Check sheet for the modelled part. Datum: model origin and axes. Units: mm. A direction names the side the tool comes from. Give positions to 0.01 mm unless a question says otherwise; leave off trailing zeros. Write each loop counter-clockwise with the first axis right and the second up, starting at its lowest first coordinate (ties: lowest second). Pieces come first, ordered by that corner, then holes. Notation, with made-up numbers: M 44.5,65 L 66.5,65 A22 ccw 66.5,101 Z; hole C 82.25,-35.5 d2. An arc over 180 degrees is marked long. Use CSV: the item, a comma, the result in double quotes. Start each with the question number.
1. Cross-section at C-C, the plane x = 3. Enter the section's corners in (y, z), and give its area (3 significant figures).
2. Depth check by flat-ended pin: P1, Ø3, axis at y = 15.5, z = 50.5, coming from the +X side (3 decimals); P2, Ø1, axis at x = 95.5, y = -12, coming from the +Z side; P3, Ø15, axis at y = -21, z = 38, coming from the -X side; P4, Ø5, axis at y = -3, z = 22.5, coming from the +X side. Enter the tip coordinate at first touch or a pass-through.
3. Scan lines: line 1 (Y direction, x = 46, z = 8); line 2 (Z direction, x = 12, y = -21); line 3 (X direction, y = -26, z = 47). Record each from-to range of solid material in increasing order.
4. Cross-section at A-A, the plane y = -21. Enter the section's corners in (x, z).
5. Mould release check, pull along Y, two halves, no side actions. Record for faces 1 (the face through (0, -21, 28)), 2 (the face through (36.5, -20.8, 9.6)), 3 (the face through (32, -42, 10)): +Y half, -Y half, draft (parallel to the pull), parting line (faces both ways), or undercut.
6. Cross-section at D-D, the plane z = 7. Enter the section's corners in (x, y), and give its area (3 significant figures).
7. Cross-section at B-B, the plane z = 39.5. Enter the section's corners in (x, y), and give its area (3 significant figures).
8. Access from +Z, -Z, +X, -X, +Y, -Y to the whole of each face (thin tool, end or side, straight path). Record for faces 4 (the face through (-6.8, 10.8, 32.1)), 5 (the face through (56.978, 10.846, 31.805)), 6 (the face through (65, -29, 19)).
from build123d import *

# Parameters (mm, degrees)
F0_W      = 42
F0_H      = 16
F1_DEPTH  = 112
F2_W      = 42
F2_H      = 22
F3_DEPTH  = 22
F4_R      = 9.5
F5_DEPTH  = 25
F6_W      = 42
F6_H      = 16
F7_DEPTH  = 21
F9_DEPTH  = 3
F11_DEPTH = 58
F13_DEPTH = 54
F15_DEPTH = 22


with BuildPart() as f1:
    # F0 (on Right) → F1 (new body)
    with BuildSketch(Plane.YZ):
        with Locations((-21, 8)):
            Rectangle(F0_W, F0_H)
    extrude(amount=F1_DEPTH)

    # F2 (on face) → F3 (join)
    with BuildSketch(Plane(origin=(0, 0, 0), x_dir=(0, -1, 0), z_dir=(-1, 0, 0))):
        with Locations((21, 27)):
            Rectangle(F2_W, F2_H)
        with BuildLine():
            ThreePointArc((42, 38), (21, 59), (0, 38))
            Line((0, 38), (42, 38))
        make_face()
    extrude(amount=-F3_DEPTH)

    # F4 (on face) → F5 (cut)
    with BuildSketch(Plane(origin=(0, 0, 0), x_dir=(0, -1, 0), z_dir=(-1, 0, 0))):
        with Locations((21, 38)):
            Circle(F4_R)
    extrude(amount=-F5_DEPTH, mode=Mode.SUBTRACT)

    # F6 (on face) → F7 (join)
    with BuildSketch(Plane(origin=(0, 0, 0), x_dir=(0, -1, 0), z_dir=(-1, 0, 0))):
        with Locations((21, 8)):
            Rectangle(F6_W, F6_H)
    extrude(amount=F7_DEPTH)

    # F8 (on face) → F9 (join)
    with BuildSketch(Plane.XY.offset(16)):
        with BuildLine():
            Line((87, -7.931874), (43, -7.931874))
            ThreePointArc((43, -7.931874), (30, -20.931874), (43, -33.931874))
            Line((43, -33.931874), (87, -33.931874))
            ThreePointArc((87, -33.931874), (100, -20.931874), (87, -7.931874))
        make_face()
    extrude(amount=F9_DEPTH)

    # F10 (on face) → F11 (cut)
    with BuildSketch(Plane.XY.offset(19)):
        with BuildLine():
            Line((87, -14.431874), (43, -14.431874))
            ThreePointArc((43, -14.431874), (36.5, -20.931874), (43, -27.431874))
            Line((43, -27.431874), (87, -27.431874))
            ThreePointArc((87, -27.431874), (93.5, -20.931874), (87, -14.431874))
        make_face()
    extrude(amount=-F11_DEPTH, mode=Mode.SUBTRACT)

    # F12 (on Top) → F13 (cut)
    with BuildSketch(Plane.XY):
        with BuildLine():
            Line((-18.401096, 0), (-17.609082, 0))
            ThreePointArc((-17.609082, 0), (-18.005089, 0.026252), (-18.401096, 0))
        make_face()
        with BuildLine():
            Line((-21, -39.485341), (-21, -38.642563))
            ThreePointArc((-21, -38.642563), (-21.029742, -39.063952), (-21, -39.485341))
        make_face()
        with BuildLine():
            ThreePointArc((-18.645877, -42), (-20.219818, -41.114213), (-21, -39.485341))
            Line((-21, -39.485341), (-21, -42))
            Line((-21, -42), (-18.645877, -42))
        make_face()
        with BuildLine():
            Line((108.139321, 0), (109.862531, 0))
            ThreePointArc((109.862531, 0), (109.000926, 0.126389), (108.139321, 0))
        make_face()
        with BuildLine():
            ThreePointArc((109.862531, 0), (111.385234, -1.052876), (112, -2.799083))
            Line((112, -2.799083), (112, 0))
            Line((112, 0), (109.862531, 0))
        make_face()
        with BuildLine():
            ThreePointArc((112, -39.063952), (111.330671, -40.953771), (109.620459, -42))
            Line((109.620459, -42), (112.000891, -42))
            Line((112.000891, -42), (112, -39.063952))
        make_face()
    extrude(amount=F13_DEPTH, mode=Mode.SUBTRACT)

    # F14 (on face) → F15 (join)
    with BuildSketch(Plane(origin=(0, 0, 0), x_dir=(-1, 0, 0), z_dir=(0, 1, 0))):
        with BuildLine():
            Line((-108.998536, 0), (11.137469, 0))
            ThreePointArc((11.137469, 0), (6.672089, 32.568119), (-6.39447, 62.732451))
            Line((-6.39447, 62.732451), (-108.998536, 0))
        make_face()
    extrude(amount=F15_DEPTH)


solid = f1.part
Worked answers:
1,outline,"M -42,0 L 22,0 L 22,56.76 L 0,56.76 L 0,38 A21 ccw -42,38 Z; hole C -21,38 d19"
1,area,"3,250 mm^2"
2,P1,"stops at x = 28.855"
2,P2,"stops at z = 19"
2,P3,"passes through"
2,P4,"stops at x = 22"
3,line 1,"y = -42 to -27.43, -14.43 to 22"
3,line 2,"z = 0 to 28.5, 47.5 to 59"
3,line 3,"x = 0 to 22"
4,outline,"M -21,0 L 36.5,0 L 36.5,19 L 30,19 L 30,16 L 22,16 L 22,28.5 L 0,28.5 L 0,16 L -21,16 Z; M 0,47.5 L 22,47.5 L 22,59 L 0,59 Z; M 93.5,0 L 112,0 L 112,16 L 100,16 L 100,19 L 93.5,19 Z"
5,face 1,"draft"
5,face 2,"undercut"
5,face 3,"-Y half"
6,outline,"M -21,-39.49 A3 ccw -18.65,-42 L 109.62,-42 A3 ccw 112,-39.06 L 112,-2.8 A3 ccw 109.86,0 L 97.55,0 L 97.55,22 L -10.93,22 L -10.93,0 L -21,0 Z; hole M 43,-27.43 L 87,-27.43 A6.5 ccw 87,-14.43 L 43,-14.43 A6.5 ccw Z"
6,area,"7,260 mm^2"
7,outline,"M -4.51,0 L 44.39,0 L 44.39,22 L -4.51,22 Z; M 0,-41.95 L 22,-41.95 L 22,-30.38 L 0,-30.38 Z; M 0,-11.62 L 22,-11.62 L 22,-0.05 L 0,-0.05 Z"
7,area,"1,580 mm^2"
8,face 4,"+Z, -X, +Y"
8,face 5,"+Z, +X, +Y"
8,face 6,"+Z, +X, -Y"
